Autodesk Fusion 360 part; units mm, degrees
sketch "Sketch1" plane through (0, 0, 0) normal (0, 0, 1) x (1, 0, 0)
  line L0 (-27, 30) -> (60, 30)
  line L1 (63, 27) -> (63, -60)
  line L2 (60, -63) -> (-27, -63)
  line L3 (-30, -60) -> (-30, 27)
  arc A0 (-27, 30) -> (-30, 27) centre (-27, 27) ccw
  arc A1 (63, 27) -> (60, 30) centre (60, 27) ccw
  arc A2 (-30, -60) -> (-27, -63) centre (-27, -60) ccw
  arc A3 (60, -63) -> (63, -60) centre (60, -60) ccw
  point P0 (-30, 30)
  point P1 (63, 30)
  point P2 (-30, -63)
  dimension "d1" = 93
  dimension "d2" = 93
  dimension "d3" = 3
  dimension "d4" = 3
extrude "Extrude1" add sketch "Sketch1" along normal blind 2
sketch "Sketch2" plane through (0, 0, 2) normal (0, 0, 1) x (-1, 0, 0)
  arc A0 (30, 60) -> (27, 63) centre (27, 60) ccw
  line L0 (27, 63) -> (-60, 63)
  arc A1 (-60, 63) -> (-63, 60) centre (-60, 60) ccw
  line L1 (-63, 60) -> (-63, -27)
  arc A2 (-63, -27) -> (-60, -30) centre (-60, -27) ccw
  line L2 (-60, -30) -> (27, -30)
  arc A3 (27, -30) -> (30, -27) centre (27, -27) ccw
  line L3 (30, -27) -> (30, 60)
  point P0 (26, -26)
  point P1 (-59, -26)
  point P2 (26, 59)
  point P3 (-60, 60)
  point P4 (-59, 59)
  point P5 (-57.2336, -24.9323)
  dimension "d18" = 85
  dimension "d19" = 4
  dimension "d20" = 4
  dimension "d21" = 4
  dimension "d22" = 4
  dimension "d23" = 4
  dimension "d24" = 4
  dimension "d25" = 85
  dimension "d26" = 4
hole "Hole2" at (59, -59, 2) at (-26, -59, 2) at (-26, 26, 2) at (59, 26, 2) direction (0, 0, -1) diameter 3 depth 2 tip angle 118
sketch "Sketch3" plane through (0, 0, 2) normal (0, 0, 1) x (-1, 0, 0)
  line L0 (-60, -30) -> (27, -30)
  line L1 (30, -27) -> (30, 60)
  line L2 (27, 63) -> (-60, 63)
  point P0 (-16.5, 16.5)
  point P1 (-16.5, -1)
  point P2 (1, 16.5)
  point P3 (-16.5, 34)
  point P4 (-34, 16.5)
  point P5 (-28.8744, 28.8744)
  point P6 (-4.1256, 28.8744)
  point P7 (-4.1256, 4.1256)
  point P8 (-28.8744, 4.1256)
  point P9 (-34, 16.5)
  point P10 (-16.5, 34)
  point P11 (1, 16.5)
  point P12 (-16.5, -1)
  point P13 (-28.8744, 4.1256)
  point P14 (-28.8744, 28.8744)
  point P15 (-4.1256, 28.8744)
  point P16 (-4.1256, 4.1256)
  point P17 (-16.5, -1)
  point P18 (-34, 16.5)
  point P19 (-16.5, 34)
  point P20 (1, 16.5)
  point P21 (-4.1256, 4.1256)
  point P22 (-28.8744, 4.1256)
  point P23 (-28.8744, 28.8744)
  point P24 (-4.1256, 28.8744)
  point P25 (1, 16.5)
  point P26 (-16.5, -1)
  point P27 (-34, 16.5)
  point P28 (-16.5, 34)
  point P29 (-4.1256, 28.8744)
  point P30 (-4.1256, 4.1256)
  point P31 (-28.8744, 4.1256)
  point P32 (-28.8744, 28.8744)
  dimension "d30" = 46.5
  dimension "d31" = 46.5
  dimension "d32" = 17.5
  dimension "d34" = 46.5
  dimension "d35" = 46.5
  dimension "d36" = 46.5
  dimension "d38" = 46.5
  dimension "d39" = 17.5
  dimension "d40" = 17.5
  dimension "d41" = 17.5
  dimension "d47" = 360
hole "Hole3" at (16.5, -34, 2) at (-1, -16.5, 2) at (16.5, 1, 2) at (34, -16.5, 2) at (16.5, -34, 2) at (4.1256, -28.8744, 2) at (4.1256, -4.1256, 2) at (28.8744, -28.8744, 2) at (28.8744, -4.1256, 2) direction (0, 0, -1) diameter 3 depth 25 tip angle 118
sketch "Sketch4" plane through (0, 0, 2) normal (0, 0, 1) x (-1, 0, 0)
sketch "Sketch5" plane through (0, 0, 2) normal (0, 0, 1) x (-1, 0, 0)
  circle A0 centre (-28.8744, 28.8744) radius 1.5
  circle A1 centre (-4.1256, 28.8744) radius 1.5
  circle A2 centre (-34, 16.5) radius 1.5
  circle A3 centre (1, 16.5) radius 1.5
  circle A4 centre (-16.5, 34) radius 1.5
  circle A5 centre (-16.5, -1) radius 1.5
  circle A6 centre (-4.1256, 4.1256) radius 1.5
  circle A7 centre (-28.8744, 4.1256) radius 1.5
  circle A8 centre (26, -26) radius 1.5
  circle A9 centre (-59, 59) radius 1.5
  circle A10 centre (26, 59) radius 1.5
  circle A11 centre (-59, -26) radius 1.5
  arc A12 (30, 60) -> (27, 63) centre (27, 60) ccw
  line L0 (27, 63) -> (-60, 63)
  arc A13 (-60, 63) -> (-63, 60) centre (-60, 60) ccw
  line L1 (-63, 60) -> (-63, -27)
  arc A14 (-63, -27) -> (-60, -30) centre (-60, -27) ccw
  line L2 (-60, -30) -> (27, -30)
  arc A15 (27, -30) -> (30, -27) centre (27, -27) ccw
  line L3 (30, -27) -> (30, 60)
  circle A16 centre (15.5, 16.5) radius 7.5
  circle A17 centre (-48.5, 16.5) radius 7.5
  dimension "d48" = 15
  dimension "d49" = 14.5
  dimension "d50" = 46.5
  dimension "d51" = 15
  dimension "d52" = 46.5
  dimension "d53" = 14.5
extrude "Extrude2" cut sketch "Sketch5" against normal blind 9 contours A16 | A17
sketch "Sketch6" plane through (0, 0, 2) normal (0, 0, 1) x (-1, 0, 0)
  circle A0 centre (-48.5, 16.5) radius 7.5
  circle A1 centre (15.5, 16.5) radius 7.5
  circle A2 centre (-28.8744, 28.8744) radius 1.5
  circle A3 centre (-4.1256, 28.8744) radius 1.5
  circle A4 centre (-34, 16.5) radius 1.5
  circle A5 centre (1, 16.5) radius 1.5
  circle A6 centre (-16.5, 34) radius 1.5
  circle A7 centre (-16.5, -1) radius 1.5
  circle A8 centre (-4.1256, 4.1256) radius 1.5
  circle A9 centre (-28.8744, 4.1256) radius 1.5
  circle A10 centre (26, -26) radius 1.5
  circle A11 centre (-59, 59) radius 1.5
  circle A12 centre (26, 59) radius 1.5
  circle A13 centre (-59, -26) radius 1.5
  arc A14 (30, 60) -> (27, 63) centre (27, 60) ccw
  line L0 (27, 63) -> (-60, 63)
  arc A15 (-60, 63) -> (-63, 60) centre (-60, 60) ccw
  line L1 (-63, 60) -> (-63, -27)
  arc A16 (-63, -27) -> (-60, -30) centre (-60, -27) ccw
  line L2 (-60, -30) -> (27, -30)
  arc A17 (27, -30) -> (30, -27) centre (27, -27) ccw
  line L3 (30, -27) -> (30, 60)
sketch "Sketch7" plane through (0, 0, 2) normal (0, 0, 1) x (-1, 0, 0)
  line L0 (19, -20) -> (2.4142, -20)
  line L1 (1.7071, -18.2929) -> (18.2929, -1.7071)
  line L2 (20, -19) -> (20, -2.4142)
  arc A0 (19, -20) -> (20, -19) centre (19, -19) ccw
  arc A1 (1.7071, -18.2929) -> (2.4142, -20) centre (2.4142, -19) ccw
  arc A2 (20, -2.4142) -> (18.2929, -1.7071) centre (19, -2.4142) ccw
  line L3 (-51.2929, 34.7071) -> (-34.7071, 51.2929)
  arc A3 (-34.7071, 51.2929) -> (-35.4142, 53) centre (-35.4142, 52) ccw
  line L4 (-52, 53) -> (-35.4142, 53)
  line L5 (-53, 52) -> (-53, 35.4142)
  arc A4 (-53, 35.4142) -> (-51.2929, 34.7071) centre (-52, 35.4142) ccw
  arc A5 (-52, 53) -> (-53, 52) centre (-52, 52) ccw
  line L6 (-60, -30) -> (27, -30)
  line L7 (-52, -20) -> (-35.4142, -20)
  arc A6 (-35.4142, -20) -> (-34.7071, -18.2929) centre (-35.4142, -19) ccw
  line L8 (-51.2929, -1.7071) -> (-34.7071, -18.2929)
  arc A7 (-51.2929, -1.7071) -> (-53, -2.4142) centre (-52, -2.4142) ccw
  line L9 (-53, -19) -> (-53, -2.4142)
  line L10 (1.7071, 51.2929) -> (18.2929, 34.7071)
  arc A8 (2.4142, 53) -> (1.7071, 51.2929) centre (2.4142, 52) ccw
  line L11 (19, 53) -> (2.4142, 53)
  arc A9 (20, 52) -> (19, 53) centre (19, 52) ccw
  line L12 (20, 52) -> (20, 35.4142)
  arc A10 (18.2929, 34.7071) -> (20, 35.4142) centre (19, 35.4142) ccw
  arc A11 (-53, -19) -> (-52, -20) centre (-52, -19) ccw
  point P0 (20, -20)
  point P1 (20, 0)
  point P2 (0, -20)
  point P3 (-52, -19)
  dimension "d56" = 1
  dimension "d61" = 1
extrude "Extrude3" cut sketch "Sketch7" against normal blind 5
sketch "Sketch8" plane through (0, 0, 0) normal (0, 0, 1) x (1, 0, 0)
  line L0 (60, 30) -> (-27, 30)
sketch "Sketch9" plane through (0, 0, 0) normal (0, 0, 1) x (1, 0, 0)
sketch "Sketch10" plane through (0, 0, 2) normal (0, 0, 1) x (-1, 0, 0)
  circle A0 centre (-17, 16.5) radius 7.5
  line L0 (-60, -30) -> (27, -30)
  dimension "d62" = 15
  dimension "d63" = 46.5
extrude "Extrude4" cut sketch "Sketch10" against normal blind 10
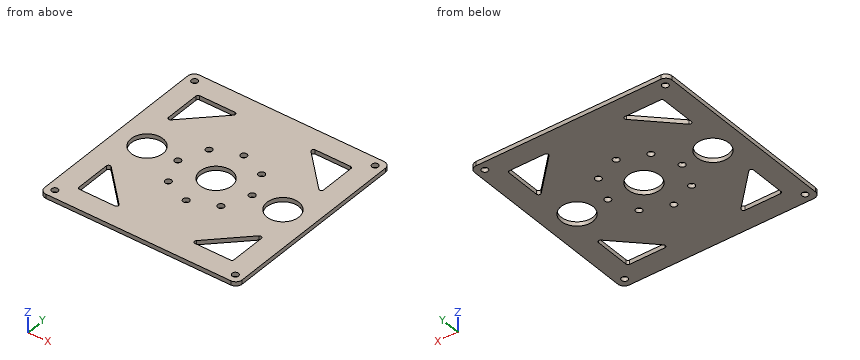
The model under review builds one solid part; all positions refer to its coordinate system, in mm. Round coordinates to 2 decimals unless told otherwise and drop trailing zeros. Loops run counter-clockwise (first coordinate to the right, second up) from the corner with the lowest first, then second, coordinate; pieces in that order, holes last. Notation, with made-up numbers: M 73.5,18 L 100.5,18 A13 cw 100.5,43 Z; hole C -22,13 d11. An arc over 180 degrees is marked long. Answer as CSV lines item,"result". Start each with the question number.
Item 1: Consider section A-A (y = -16.5). Write out the cut boundary in (x, z), then the cut area to 3 significant figures.
Item 2: Wall thickness on line 1 (Y direction, x = -1, z = 0.65); line 2 (X direction, y = -16.5, z = 0.9); line 3 (X direction, y = -43, z = 0.9): over which ranges is each line inside the solid? List them lowest first. Write a range as [from, to].
Item 3: Consider section B-B (x = -15.5). Write out the cut boundary in (y, z).
Item 4: Consider section C-C (y = 5.5). Write out the cut boundary in (x, z).
Item 5: Consider section D-D (x = 23). Write out the cut boundary in (y, z).
Item 6: Insertion check: P1, Ø1.8, axis at x = 4.13, y = -28.87, coming from the -Z side (3 decimals). The pin has a flat end and moves straight along its axis. Give the tip position at first contact, or say it passes through.
Answer:
1,outline,"M -30,0 L -23,0 L -23,2 L -30,2 Z; M -8,0 L -2.5,0 L -2.5,2 L -8,2 Z; M 0.5,0 L 9.5,0 L 9.5,2 L 0.5,2 Z; M 24.5,0 L 32.5,0 L 32.5,2 L 24.5,2 Z; M 35.5,0 L 41,0 L 41,2 L 35.5,2 Z; M 56,0 L 63,0 L 63,2 L 56,2 Z"
1,area,"84.0 mm^2"
2,line 1,"y = [-63, -18], [-15, 30]"
2,line 2,"x = [-30, -23], [-8, -2.5], [0.5, 9.5], [24.5, 32.5], [35.5, 41], [56, 63]"
2,line 3,"x = [-30, -20], [-10, 43], [53, 63]"
3,outline,"M -63,0 L -53,0 L -53,2 L -63,2 Z; M -37.5,0 L -24,0 L -24,2 L -37.5,2 Z; M -9,0 L 4.5,0 L 4.5,2 L -9,2 Z; M 20,0 L 30,0 L 30,2 L 20,2 Z"
4,outline,"M -30,0 L -20,0 L -20,2 L -30,2 Z; M -14.5,0 L 47.5,0 L 47.5,2 L -14.5,2 Z; M 53,0 L 63,0 L 63,2 L 53,2 Z"
5,outline,"M -63,0 L -21,0 L -21,2 L -63,2 Z; M -12,0 L 30,0 L 30,2 L -12,2 Z"
6,P1,"passes through"
